```python
from build123d import *

# Parameters (mm, degrees)
SKETCH066_W             = 50
SKETCH066_H             = 20
PAD065_DEPTH            = 5
SKETCH067_W             = 50
SKETCH067_H             = 3
PAD066_DEPTH            = 20
SKETCH068_W             = 50
SKETCH068_H             = 10
PAD067_DEPTH            = 3
BODY046_ROLL_ANGLE      = 90
BODY046_PITCH_ANGLE     = -60
BODY046_PLACEMENT_ANGLE = -90


with BuildPart() as part:
    # Sketch066 → Pad065 (new body)
    with BuildSketch(Plane.XY):
        with Locations((184.845276, -123.914059)):
            Rectangle(SKETCH066_W, SKETCH066_H)
    extrude(amount=PAD065_DEPTH)

    # Sketch067 (on Face6 of Pad065) → Pad066 (join)
    with BuildSketch(Plane.XY.offset(5)):
        with Locations((184.83606, -132.417099)):
            Rectangle(SKETCH067_W, SKETCH067_H)
    extrude(amount=PAD066_DEPTH)

    # Sketch068 (on Face7 of Pad066) → Pad067 (join)
    with BuildSketch(Plane(origin=(0, -113.914059, 0), x_dir=(-1, 0, 0), z_dir=(0, 1, 0))):
        with Locations((-184.841869, 9.989668)):
            Rectangle(SKETCH068_W, SKETCH068_H)
    extrude(amount=-PAD067_DEPTH)


with BuildPart() as part_1:
    # Body046 roll: moved
    add(part.part.rotate(Axis((0, 0, 0), (1, 0, 0)), BODY046_ROLL_ANGLE))


with BuildPart() as part_2:
    # Body046 pitch: moved
    add(part_1.part.rotate(Axis((0, 0, 0), (0, 1, 0)), BODY046_PITCH_ANGLE))


with BuildPart() as part_3:
    # Body046 placement: moved
    add(part_2.part.moved(Location((125.51314, 216.468461, 42.886067))).rotate(Axis((125.51314, 216.468461, 42.886067), (0, 0, 1)), BODY046_PLACEMENT_ANGLE))


solid = part_3.part
```
Verification items for the finished model (mm, model axes). A direction names the side the tool comes from. Round coordinates to 2 decimals unless told otherwise and drop trailing zeros. Write each loop counter-clockwise with the first axis right and the second up, starting at its lowest first coordinate (ties: lowest second). Pieces come first, ordered by that corner, then holes. Notation, with made-up numbers: (70, -11.5) - (88, -11.5) arc R12 ccw to (88, 5.5) - close; hole circle Ø9 at (22.5, 28). An arc over 180 degrees is marked (long way). Answer as a JSON object with one key per item and string values. Group by question number.
Q1. Go/stop test with flat-tipped pins: pin 1 Ø2 at (x, y) = (113.5, 0) entering from +Z; pin 2 Ø4 at (x, z) = (121.5, 131) entering from +Y; pin 3 Ø22 at (y, z) = (22.5, 155) entering from -X. Record where each tip stops, or that it passes through.
Q2. Tool access check on faces 1 (the flat face through (118.123, 25.569, 145.705)), 2 (the flat face through (110.523, 24, 146)), 3 (the flat face through (120.513, 17, 141)). Record the directions out of +Z, -Z, +X, -X, +Y, -Y that give a thin tool (end or side, any length) a straight path to the whole face; none if there is none.
Q3. Mould release check, pull along Z, two halves, no side actions. Record for faces 4 (the flat face through (115.588, 11.614, 166.918)), 5 (the flat face through (100.513, 10, 136)), 6 (the flat face through (110.653, 10.848, 137.197)): released by +Z, released by -Z, zero draft, split by the parting line, or undercut.
Q4. Thickness scan on line 1 (X direction, y = 13.5, z = 157); line 2 (Y direction, x = 112.75, z = 144); line 3 (Y direction, x = 115.25, z = 134). Record the ranges inside material, lowest first.
Q5. Section check A-A, the plane x = 113. Enter the section's corners in (y, z), plus the area to 3 significant figures.
Q6. Section check D-D, the plane x = 102.5. Enter the section's corners in (y, z).
Found:
{
 "1": {"pin 1": "stops at z = 157.72", "pin 2": "stops at y = 35.21", "pin 3": "stops at x = 110.52"},
 "2": {"face 1": "+Z, +X, -X, +Y", "face 2": "+Z, -X, +Y", "face 3": "-X"},
 "3": {"face 4": "released by +Z", "face 5": "zero draft", "face 6": "undercut"},
 "4": {"line 1": "x = 120.51 to 125.51", "line 2": "y = 3.46 to 6.92, 23.09 to 26.55", "line 3": "y = 9.23 to 12.69, 28.86 to 32.33"},
 "5": {"outline": "(-4.43, 157.65) - (20.57, 114.35) - (23.17, 115.85) - (-1.83, 159.15) - close; (10.3, 166.16) - (35.3, 122.86) - (37.9, 124.36) - (12.9, 167.66) - close", "area": "300 mm^2"},
 "6": {"outline": "(-4.43, 157.65) - (20.57, 114.35) - (23.17, 115.85) - (-1.83, 159.15) - close"}
}
